Design review of the part built by this model. Coordinates are the model's own, in mm. A direction names the side the tool comes from. Coordinates: 2 decimals unless noted, no trailing zeros. Loops run counter-clockwise (first coordinate to the right, second up) from the corner with the lowest first, then second, coordinate; pieces in that order, holes last. Notation, with made-up numbers: M 46,-18 L 57,-18 A21 ccw 57,2 Z; hole C 71.25,41 d6. An arc over 180 degrees is marked long. One line per item, written item: value.
```python
from build123d import *

# Parameters (mm, degrees)
F0_W     = 490
F0_H     = 460
F0_W_2   = 410
F0_H_2   = 40
F1_DEPTH = 40
F2_W     = 40
F2_H     = 40
F3_DEPTH = 623
F4_W     = 290
F4_H     = 40
F4_W_2   = 330
F5_DEPTH = 40
F6_W     = 220
F6_H     = 40
F7_DEPTH = 40
F8_W     = 220
F8_H     = 40
F9_DEPTH = 40


with BuildPart() as f1:
    # F0 (on Top) → F1 (new body)
    with BuildSketch(Plane.XY):
        Rectangle(F0_W, F0_H)
        Polygon((205, -150), (205, -190), (-205, -190), (-205, -150), (-205, -110), (-205, 110), (-205, 150), (-205, 190), (205, 190), (205, 150), (205, 110), (205, -110), align=None, mode=Mode.SUBTRACT)
        with Locations((0, 130)):
            Rectangle(F0_W_2, F0_H_2)
        with Locations((0, -130)):
            Rectangle(F0_W_2, F0_H_2)
    extrude(amount=F1_DEPTH)

    # F2 (on face) → F3 (join)
    with BuildSketch(Plane.XY.offset(40)):
        with Locations((-145, 130)):
            Rectangle(F2_W, F2_H)
        with Locations((145, 130)):
            Rectangle(F2_W, F2_H)
        with Locations((145, -130)):
            Rectangle(F2_W, F2_H)
        with Locations((-145, -130)):
            Rectangle(F2_W, F2_H)
    extrude(amount=F3_DEPTH)

    # F4 (on face) → F5 (join)
    with BuildSketch(Plane.XY.offset(663)):
        with Locations((-20, 130)):
            Rectangle(F4_W, F4_H)
        with Locations((0, -130)):
            Rectangle(F4_W_2, F4_H)
    extrude(amount=-F5_DEPTH)

    # F6 (on face) → F7 (join)
    with BuildSketch(Plane.YZ.offset(165)):
        with Locations((0, 351.5)):
            Rectangle(F6_W, F6_H)
    extrude(amount=-F7_DEPTH)

    # F8 (on face) → F9 (join)
    with BuildSketch(Plane(origin=(-165, 0, 0), x_dir=(0, -1, 0), z_dir=(-1, 0, 0))):
        with Locations((0, 351.5)):
            Rectangle(F8_W, F8_H)
    extrude(amount=-F9_DEPTH)


solid = f1.part
```
(1) To check wall thickness, follow line 1 along Y through (x, z) = (-182, 34.5); line 2 along X through (y, z) = (-146.5, 470); line 3 along Z through (x, y) = (10, 115). State the ranges of each line that lie inside material, in increasing order. Write a range as [from, to].
Reply:
line 1: y = [-230, -190], [-150, -110], [110, 150], [190, 230]
line 2: x = [-165, -125], [125, 165]
line 3: z = [0, 40], [623, 663]
(2) We need section D-D on x = 88. State the section outline as (y, z) points.
Reply:
outline: M -230,0 L -190,0 L -190,40 L -230,40 Z; M -150,0 L -110,0 L -110,40 L -150,40 Z; M -150,623 L -110,623 L -110,663 L -150,663 Z; M 110,0 L 150,0 L 150,40 L 110,40 Z; M 110,623 L 150,623 L 150,663 L 110,663 Z; M 190,0 L 230,0 L 230,40 L 190,40 Z
(3) Mouldability with a two-part tool opening along Z and no side actions: class faces 6 (the flat face through (-2, 130, 623)), 7 (the flat face through (-2, 130, 663)), 8 (the flat face through (-3, 230, 20)) as released by +Z, released by -Z, zero draft, split by the parting line, or undercut.
Reply:
face 6: undercut
face 7: released by +Z
face 8: zero draft
(4) We need section B-B on z = 402.5. State the section outline as (x, y) points, then the cut area to 3 significant figures.
Reply:
outline: M -165,-150 L -125,-150 L -125,-110 L -165,-110 Z; M -165,110 L -125,110 L -125,150 L -165,150 Z; M 125,-150 L 165,-150 L 165,-110 L 125,-110 Z; M 125,110 L 165,110 L 165,150 L 125,150 Z
area: 6,400 mm2
(5) Insertion check: pin 1 (3 mm diameter, centred on y = 125.5, z = 141, fed in from +X); pin 2 (6 mm diameter, centred on x = 154, y = -14, fed in from +Z); pin 3 (20 mm diameter, centred on x = -140.5, y = 18, fed in from -Z). Each pin has a flat end and moves straight along its axis. Give the tip position at first contact, or say it passes through.
Reply:
pin 1: stops at x = 165
pin 2: stops at z = 371.5
pin 3: stops at z = 331.5
(6) We need section C-C on x = 157. State the section outline as (y, z) points.
Reply:
outline: M -230,0 L -190,0 L -190,40 L -230,40 Z; M -150,0 L -110,0 L -110,331.5 L 110,331.5 L 110,0 L 150,0 L 150,663 L 110,663 L 110,371.5 L -110,371.5 L -110,663 L -150,663 Z; M 190,0 L 230,0 L 230,40 L 190,40 Z
(7) Tool access review of faces 1 (the flat face through (24, -110, 625)), 2 (the flat face through (205, -170, 20)), 3 (the flat face through (-2, -130, 623)), 4 (the flat face through (-145, 2, 331.5)), 5 (the flat face through (-1, 110, 30)): name each direction out of +Z, -Z, +X, -X, +Y, -Y from which nothing blocks a thin tool from reaching the whole face with its end or side.
Reply:
face 1: +Z, +X, -X
face 2: +Z, -Z
face 3: +Y, -Y
face 4: -Z, +X, -X
face 5: -Z
(8) We need section A-A on y = 17.5. State the section outline as (x, z) points, then the cut area to 3 significant figures.
Reply:
outline: M -245,0 L -205,0 L -205,40 L -245,40 Z; M -165,331.5 L -125,331.5 L -125,371.5 L -165,371.5 Z; M 125,331.5 L 165,331.5 L 165,371.5 L 125,371.5 Z; M 205,0 L 245,0 L 245,40 L 205,40 Z
area: 6,400 mm2
